CAD build for the part. Positions are in the model's coordinates, mm. A direction names the side the tool comes from. Coordinates: 2 decimals unless noted, no trailing zeros. Write each loop counter-clockwise with the first axis right and the second up, starting at its lowest first coordinate (ties: lowest second). Pieces come first, ordered by that corner, then holes. Notation, with made-up numbers: (33.5, -36.5) - (39.5, -36.5) arc R27 ccw to (39.5, -10.5) - close; hole circle Ø11 at (59, -10). An arc over 180 degrees is marked (long way). Answer in a Markdown table with one row per item. Add a question column.
Q1. Two-plate mould, pull along Z, no slides. Class faces 6 (the flat face through (0, -1, 1.5)), 7 (the flat face through (0, -4, 6)), 8 (the flat face through (-0.1, 0, -3.6)), 9 (the flat face through (0, -3.5, 0)): +Z half, -Z half, draft (parallel to the pull), parting line (faces both ways), or undercut.
Q2. Pin check, flat tip, straight feed: pin 1 (2 mm diameter, centred on y = 0, z = 3, fed in from -X). Stop position of the tip, or through.
Q3. Band-saw the part on D-D (x = -3.25). State how many separate pieces and enclosed holes the cut face has, and give its area (3 significant figures).
Q4. Band-saw the part on A-A (y = -1.75). List the corners of the cut face in (x, z).
Q5. Drill centre lines: line 1 along X through (y, z) = (-2.75, 2); line 2 along Y through (x, z) = (3.75, 1.5); line 3 along Z through (x, y) = (-1.75, -1.75). Where is each one in solid material? Low to high. Write a range as from..to.
Q6. Band-saw the part on B-B (x = 4). List the corners of the cut face in (y, z).
Q7. Band-saw the part on C-C (z = -0.5). List the corners of the cut face in (x, y), and give its area (3 significant figures).
Q8. 3-axis set-ups, long thin cutter, end or side, ignore diameter. For faces 1 (the flat face through (0, 1.5, 2)), 2 (the flat face through (0, 0, 3.6)), 3 (the flat face through (-4.994, -4, 0)), 4 (the cylindrical face through (0, -1.7, -3.2)), 5 (the flat face through (0, -1, -1.5)): which of +Z, -Z, +X, -X, +Y, -Y reach the whole face in a straight line?
Autodesk Inventor part; units mm, degrees
ref_plane "YZ Plane" through (0, 0, 0) normal (1, 0, 0) x (0, 1, 0)
ref_plane "XZ Plane" through (0, 0, 0) normal (0, 1, 0) x (-1, 0, 0)
ref_plane "XY Plane" through (0, 0, 0) normal (0, 0, 1) x (1, 0, 0)
sketch "Sketch1" plane through (0, 0, 0) normal (0, 0, 1) x (1, 0, 0)
  line L0 (0, 4) -> (0, 0)
  line L1 (0, 0) -> (4, 0)
  line L2 (4, 0) -> (0, 4)
  dimension "d45" = 4
  dimension "d46" = 4
revolve "Revolution1" add sketch "Sketch1" angle 360 about axis through (0, 4, 0) along (0, -1, 0)
sketch "Sketch2" plane through (0, 0, 0) normal (0, -1, 0) x (1, 0, 0)
  circle A0 centre (0, 0) radius 3.2
  point P0 (0, 0)
  dimension "d3" = 6.4
extrude "Extrusion1" add sketch "Sketch2" along normal blind 3.5
sketch "Sketch3" plane through (0, -3.5, 0) normal (0, -1, 0) x (1, 0, 0)
  circle A0 centre (0, 0) radius 4
  line L0 (-4.5, 1.5) -> (4.5, 1.5)
  line L1 (4.5, 1.5) -> (4.5, -1.5)
  line L2 (4.5, -1.5) -> (-4.5, -1.5)
  line L3 (-4.5, -1.5) -> (-4.5, 1.5)
  point P0 (0, 0)
  point P1 (0, 1.5)
  point P2 (4.5, 0)
  dimension "d27" = 0.5
  dimension "d28" = 3
extrude "Extrusion2" cut sketch "Sketch3" against normal through all contours A0 L2 L0 | A0 L0 L1 L2 | A0 L2 L3 L0
sketch "Sketch4" plane through (0, -3.5, 0) normal (0, -1, 0) x (1, 0, 0)
  line L0 (4.9945, 6) -> (-4.9945, 6)
  line L1 (-4.9945, 6) -> (-4.9945, -6)
  line L2 (-4.9945, -6) -> (4.9945, -6)
  line L3 (4.9945, -6) -> (4.9945, 6)
  arc A0 (-1.5, 3.7021) -> (-1.5, -3.7021) centre (0, 0) ccw
  arc A1 (-1.5, 3.4857) -> (-1.5, -3.4857) centre (0, 0) ccw
  line L4 (-1.5, 3.4857) -> (-1.5, 3.7021)
  line L5 (-1.5, -3.7021) -> (-1.5, -3.4857)
  arc A2 (-3.7081, -1.5) -> (3.7081, -1.5) centre (0, 0) ccw
  point P0 (4.9945, 0)
  point P1 (0, -6)
  point P2 (4.7697, 1.5)
  point P3 (-4.7697, 1.5)
  dimension "d18" = 1
  dimension "d42" = 1
extrude "Extrusion3" add sketch "Sketch4" along normal blind 1 contours L3 L2 L1 L0 | L4 A1 L5 A0
sketch "Sketch9" plane through (4.9945, -3.5, 6) normal (1, 0, 0) x (0, 0, -1)
  line L0 (3.5, 6) -> (8.5, 6)
  line L1 (8.5, 6) -> (8.5, 5)
  line L2 (8.5, 5) -> (3.5, 5)
  line L3 (3.5, 5) -> (3.5, 6)
  line L4 (4.5, 6) -> (2, 3.5)
  line L5 (4.9945, 3.5) -> (4.9945, 6)
  line L6 (4.9945, 3.5) -> (4.9945, 2.5)
  line L7 (7.5, 6) -> (10, 3.5)
  point P0 (6, 3.5)
  point P1 (4.5, 3.5)
  point P2 (7.5, 3.5)
  point P3 (10, 3.5)
  dimension "d47" = 1
extrude "Extrusion8" cut sketch "Sketch9" against normal through all
equation "\"d46\" = d45"
equation "\"d27\" = d22"
equation "\"d28\" = d19"
equation "\"d42\" = d18"
properties part number "Snap"
Checked values:
| question | item | result |
|---|---|---|
| 1 | face 6 | undercut |
| 1 | face 7 | +Z half |
| 1 | face 8 | draft |
| 1 | face 9 | undercut |
| 2 | pin 1 | stops at x = -3.46 |
| 3 | separate pieces | 3 |
| 3 | enclosed holes | 0 |
| 3 | area | 12.4 mm² |
| 4 | outline | (-2.83, -1.5) arc R3.2 ccw to (2.83, -1.5) - close; (-2.83, 1.5) - (2.83, 1.5) arc R3.2 ccw to start |
| 5 | line 1 | x = -2.5..2.5 |
| 5 | line 2 | y = -4.5..-3.5 |
| 5 | line 3 | z = -2.68..-1.5, 1.5..2.68 |
| 6 | outline | (-4.5, -6) - (-3.5, -6) - (-3.5, 6) - (-4.5, 6) - close |
| 7 | outline | (-4.99, -4.5) - (4.99, -4.5) - (4.99, -3.5) - (-4.99, -3.5) - close |
| 7 | area | 9.99 mm² |
| 8 | face 1 | +Z, -Z, +X, -X, +Y |
| 8 | face 2 | +Z |
| 8 | face 3 | +Z, -Z, -X, +Y, -Y |
| 8 | face 4 | -Z |
| 8 | face 5 | +X, -X, +Y |
